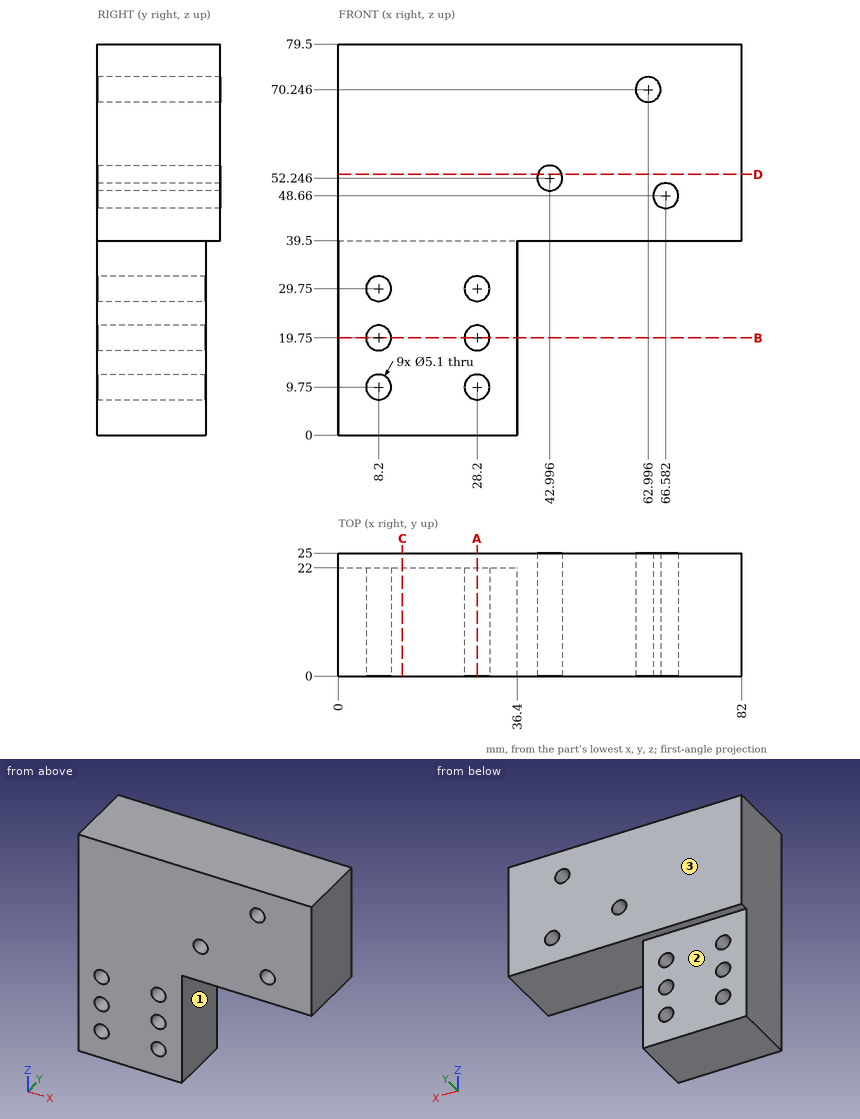
Input: dimensioned drawing with shaded views. Units: mm. Origin: part minimum x, y, z. A direction names the side the tool comes from. Give positions to 0.01 mm unless a question says otherwise; leave off trailing zeros. Write each loop counter-clockwise with the first axis right and the second up, starting at its lowest first coordinate (ties: lowest second). Pieces come first, ordered by that corner, then holes.
Q1. Set-up query: the marked faces 1, 2 and 3. Return all of +Z, -Z, +X, -X, +Y, -Y with unobstructed straight access to the full face (end or side cutting, diameter ignored); none if empty.
Q2. Section C-C, the plane x = 13. Output: boundary loops of the cut face in (y, z).
Q3. Section D-D, the plane z = 53. Output: boundary loops of the cut face in (x, y).
Q4. Section A-A, the plane x = 28.2. Output: boundary loops of the cut face in (y, z).
Q5. Material intervals for probe 1 along X at (y, z) = (12, 9.75); probe 2 along Z at (x, y) = (63, 1.75) (1 decimal); probe 3 along Y at (x, z) = (6, 11.5), sorted ascending.
Q6. First-contact query: P1, Ø4, axis at x = 28.2, z = 19.75, coming from the +Y side; P2, Ø3, axis at x = 38, y = 9, coming from the -Z side; P3, Ø11, axis at x = 22, z = 23.5, coming from the +Y side. Flat tips, straight axial feed; report the tip coordinate or a pass-through.
Q7. Section B-B, the plane z = 19.75. Output: boundary loops of the cut face in (x, y).
Filled in:
1. face 1: -Z, +X, +Y, -Y
1. face 2: -Z, +X, -X, +Y
1. face 3: +Z, -Z, +X, -X, +Y
2. outline: (0, 0) - (22, 0) - (22, 39.5) - (25, 39.5) - (25, 79.5) - (0, 79.5) - close
3. outline: (0, 0) - (40.56, 0) - (40.56, 25) - (0, 25) - close; (45.43, 0) - (82, 0) - (82, 25) - (45.43, 25) - close
4. outline: (0, 0) - (22, 0) - (22, 7.2) - (0, 7.2) - close; (0, 12.3) - (22, 12.3) - (22, 17.2) - (0, 17.2) - close; (0, 22.3) - (22, 22.3) - (22, 27.2) - (0, 27.2) - close; (0, 32.3) - (22, 32.3) - (22, 39.5) - (25, 39.5) - (25, 79.5) - (0, 79.5) - close
5. probe 1: x = 0 to 5.65, 10.75 to 25.65, 30.75 to 36.4
5. probe 2: z = 39.5 to 67.7, 72.8 to 79.5
5. probe 3: y = 0 to 22
6. P1: passes through
6. P2: stops at z = 39.5
6. P3: stops at y = 22
7. outline: (0, 0) - (5.65, 0) - (5.65, 22) - (0, 22) - close; (10.75, 0) - (25.65, 0) - (25.65, 22) - (10.75, 22) - close; (30.75, 0) - (36.4, 0) - (36.4, 22) - (30.75, 22) - close
